Geometry check sheet. Reference: the model listing, model coordinates, mm. Face numbers are marked on the shaded views. A direction names the side the tool comes from. Give positions to 0.01 mm unless a question says otherwise; leave off trailing zeros. Write each loop counter-clockwise with the first axis right and the second up, starting at its lowest first coordinate (ties: lowest second). Pieces come first, ordered by that corner, then holes. Notation, with made-up numbers: M 21.25,28.25 L 30.25,28.25 A4 cw 30.25,32.25 Z; hole C 28.5,68 d3. An arc over 180 degrees is marked long. Use one line per item in the form item = value. Start each with the question number.
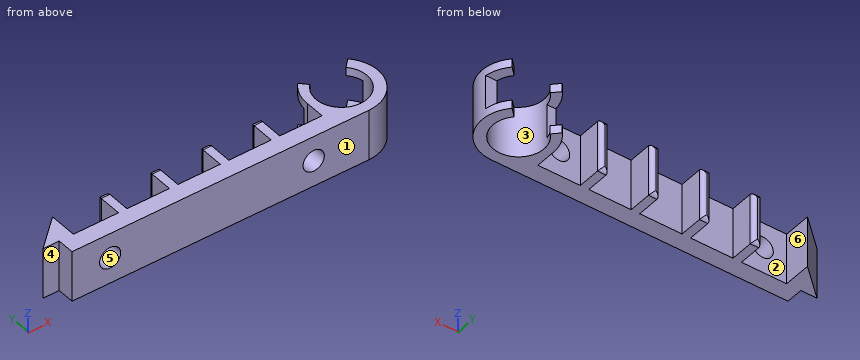
```python
from build123d import *

# Parameters (mm, degrees)
BOSS_EXTRU_1_DEPTH      = 12
ESQUISSE2_R             = 6
ENL_V_MAT_EXTRU_1_DEPTH = 12
ESQUISSE5_W             = 22.19086736
ESQUISSE5_H             = 9.756409295
ENL_V_MAT_EXTRU_2_DEPTH = 8
ENL_V_MAT_EXTRU_3_DEPTH = 60.309125122
CONG_1_R                = 1
ESQUISSE7_R             = 2.5
ENL_V_MAT_EXTRU_4_DEPTH = 4


with BuildPart() as part:
    # Esquisse1 → Boss.-Extru.1 (new body)
    with BuildSketch(Plane.XY):
        with BuildLine():
            Line((-48.320645407, 10.526434737), (-55.480460412, 4.026434737))
            Line((-55.480460412, 4.026434737), (-51.660830402, 4.026434737))
            Line((-51.660830402, 4.026434737), (-51.660830402, 0.026434737))
            Line((-51.660830402, 0.026434737), (18.339169598, 0.026434737))
            ThreePointArc((18.339169598, 0.026434737), (26.920875662, 8.608140801), (18.339169598, 17.189846865))
            ThreePointArc((18.339169598, 17.189846865), (12.553618084, 14.559253744), (10.32272561, 8.608140801))
            Line((10.32272561, 8.608140801), (10.32272561, 4.026434737))
            Line((10.32272561, 4.026434737), (0.32272561, 4.026434737))
            Line((0.32272561, 4.026434737), (0.32272561, 10.398479958))
            Line((0.32272561, 10.398479958), (-1.67727439, 10.398479958))
            Line((-1.67727439, 10.398479958), (-1.67727439, 4.026434737))
            Line((-1.67727439, 4.026434737), (-11.67727439, 4.026434737))
            Line((-11.67727439, 4.026434737), (-11.67727439, 10.398479958))
            Line((-11.67727439, 10.398479958), (-13.67727439, 10.398479958))
            Line((-13.67727439, 10.398479958), (-13.67727439, 4.026434737))
            Line((-13.67727439, 4.026434737), (-23.67727439, 4.026434737))
            Line((-23.67727439, 4.026434737), (-23.67727439, 10.398479958))
            Line((-23.67727439, 10.398479958), (-25.67727439, 10.398479958))
            Line((-25.67727439, 10.398479958), (-25.67727439, 4.026434737))
            Line((-25.67727439, 4.026434737), (-35.67727439, 4.026434737))
            Line((-35.67727439, 4.026434737), (-35.67727439, 10.398479958))
            Line((-35.67727439, 10.398479958), (-37.67727439, 10.398479958))
            Line((-37.67727439, 10.398479958), (-37.67727439, 4.026434737))
            Line((-37.67727439, 4.026434737), (-44.980460412, 4.026434737))
            Line((-44.980460412, 4.026434737), (-48.320645407, 4.026434737))
            Line((-48.320645407, 4.026434737), (-48.320645407, 10.526434737))
        make_face()
    extrude(amount=BOSS_EXTRU_1_DEPTH)

    # Esquisse2 → Enlèv. mat.-Extru.1 (cut)
    with BuildSketch(Plane.XY.offset(12)):
        with Locations((18.339169598, 8.608140801)):
            Circle(ESQUISSE2_R)
    extrude(amount=-ENL_V_MAT_EXTRU_1_DEPTH, mode=Mode.SUBTRACT)

    # Esquisse5 → Enlèv. mat.-Extru.2 (cut)
    with BuildSketch(Plane.XY.offset(2)):
        with Locations((18.196730475, 14.519832028)):
            Rectangle(ESQUISSE5_W, ESQUISSE5_H)
    extrude(amount=ENL_V_MAT_EXTRU_2_DEPTH, mode=Mode.SUBTRACT)

    # Esquisse6 → Enlèv. mat.-Extru.3 (cut, through all)
    with BuildSketch(Plane.XY):
        Polygon((6.09054696, 20.904289339), (18.339169598, 8.608140801), (30.683028441, 20.904289339), align=None)
    extrude(amount=ENL_V_MAT_EXTRU_3_DEPTH, mode=Mode.SUBTRACT)

    # Congé1
    cong_1_edges = [part.edges().sort_by_distance(p)[0] for p in [
        (-36.67727439, 10.398479958, 0),
        (-0.67727439, 10.398479958, 12),
        (-24.67727439, 10.398479958, 0),
        (-12.67727439, 10.398479958, 0),
        (-0.67727439, 10.398479958, 0),
        (-12.67727439, 10.398479958, 12),
        (-37.67727439, 10.398479958, 6),
        (-35.67727439, 10.398479958, 6),
        (-25.67727439, 10.398479958, 6),
        (-23.67727439, 10.398479958, 6),
        (-13.67727439, 10.398479958, 6),
        (-11.67727439, 10.398479958, 6),
        (-1.67727439, 10.398479958, 6),
        (0.32272561, 10.398479958, 6),
        (-24.67727439, 10.398479958, 12),
        (-36.67727439, 10.398479958, 12),
    ]]
    fillet(cong_1_edges, radius=CONG_1_R - 0.0001)  # a hair under: the kernel refuses the full size

    # Esquisse7 → Enlèv. mat.-Extru.4 (cut)
    with BuildSketch(Plane(origin=(0, 4.026434737, 0), x_dir=(1, 0, 0), z_dir=(0, 1, 0))):
        with Locations(Location((-42.67727439, -6.1321655, 0), (0, 0, 180))):
            Circle(ESQUISSE7_R)
        with Locations(Location((5.32272561, -6.1321655, 0), (0, 0, 180))):
            Circle(ESQUISSE7_R)
    extrude(amount=-ENL_V_MAT_EXTRU_4_DEPTH, mode=Mode.SUBTRACT)


solid = part.part
```
(1) Sectioned sample at A-A, the plane y = 11.5. Record the boundary of the cut face in (x, z).
(2) Sectioned sample at D-D, the plane z = 7.5. State how many separate pieces and enclosed holes the cut face has, plus the area to 3 significant figures.
(3) Sectioned sample at B-B, the plane y = 5.75. Record the boundary of the cut face in (x, z), plus the area to 3 significant figures.
(4) Tool access check on the marked faces 4, 5 and 6. Record the directions out of +Z, -Z, +X, -X, +Y, -Y that give a thin tool (end or side, any length) a straight path to the whole face; none if there is none.
(5) Sectioned sample at C-C, the plane x = -46. Record the boundary of the cut face in (y, z), plus the area to 3 significant figures.
(6) Depth check by flat-ended pin: pin 1 (1.1 mm diameter, centred on x = -52.5, z = 8.5, fed in from -Y); pin 2 (1 mm diameter, centred on x = 11.5, z = 5, fed in from +Y); pin 3 (3 mm diameter, centred on x = -44, z = 4.5, fed in from -Y); pin 4 (2.5 mm diameter, centred on y = 6, z = 8, fed in from +X). Enter the tip coordinate at first touch or a pass-through.
(7) Thickness scan on probe 1 along Y at (x, z) = (-45.5, 9); probe 2 along Y at (x, z) = (21.5, 2); probe 3 along X at (y, z) = (2.5, 11.5). Record the ranges inside material, lowest first. Write a range as [from, to].
(8) Draft check along Y on the marked faces 1, 2 and 3. Enter one of: released by +Y, released by -Y, zero draft, split by the parting line, or undercut.
Numbers:
q1.outline = M 10.74,0 L 13.08,0 L 13.08,2 L 10.74,2 Z; M 10.74,10 L 13.08,10 L 13.08,12 L 10.74,12 Z; M 23.6,0 L 26.42,0 L 26.42,2 L 23.6,2 Z; M 23.6,10 L 26.42,10 L 26.42,12 L 23.6,12 Z
q2.separate_pieces = 3
q2.enclosed_holes = 0
q2.area = 362 mm2
q3.outline = M -53.58,0 L -48.32,0 L -48.32,12 L -53.58,12 Z; M -37.68,0 L -35.68,0 L -35.68,12 L -37.68,12 Z; M -25.68,0 L -23.68,0 L -23.68,12 L -25.68,12 Z; M -13.68,0 L -11.68,0 L -11.68,12 L -13.68,12 Z; M -1.68,0 L 0.32,0 L 0.32,12 L -1.68,12 Z; M 10.32,0 L 13.06,0 L 13.06,12 L 10.32,12 Z; M 23.61,0 L 26.43,0 L 26.43,12 L 23.61,12 Z
q3.area = 226 mm2
q4.face_4 = +Z, -Z, -X, -Y
q4.face_5 = +Y, -Y
q4.face_6 = +Z, -Z, +Y
q5.outline = M 0.03,0 L 4.03,0 L 4.03,12 L 0.03,12 Z
q5.area = 48.0 mm2
q6.pin_1 = 4.03
q6.pin_2 = 9.64
q6.pin_3 = 0.03
q6.pin_4 = 26.81
q7.probe_1 = [0.03, 4.03]
q7.probe_2 = [0.63, 3.51]
q7.probe_3 = [-51.66, 24.37]
q8.face_1 = released by -Y
q8.face_2 = released by +Y
q8.face_3 = undercut
